Print and shaded views of the part. All mm, measured from the part's lowest x, y and z. Round coordinates to 2 decimals unless told otherwise and drop trailing zeros. Loops run counter-clockwise (first coordinate to the right, second up) from the corner with the lowest first, then second, coordinate; pieces in that order, holes last. Notation, with made-up numbers: (42.25, 84) - (73.25, 84) arc R21 ccw to (73.25, 108) - close; hole circle Ø9 at (27.25, 69). An arc over 180 degrees is marked (long way). Use one line per item in the form item = value.
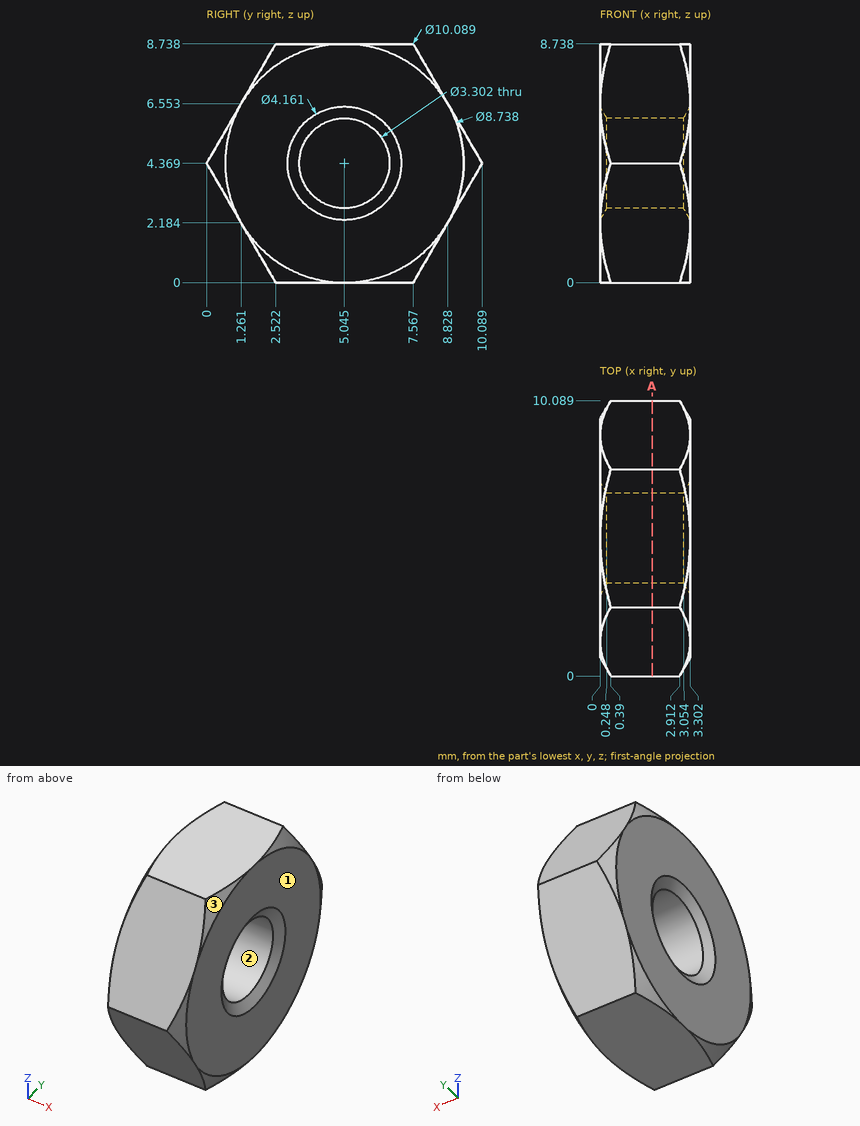
1. Flat gauge pins, fed straight in: pin 1 (1.5 mm diameter, centred on x = 3, z = 1, fed in from -Y); pin 2 (1.5 mm diameter, centred on x = 2, z = 7.5, fed in from +Y) (1 decimal). Where does each tip first touch, or does it go through?
Geometry check:
pin_1 = 1.51
pin_2 = 8.7
2. Pull direction Z, two halves, no side cores. Call the marked faces 1, 2 and 3: +Z half, -Z half, draft (parallel to the pull), parting line (faces both ways), or undercut.
Geometry check:
face_1 = draft
face_2 = undercut
face_3 = +Z half
3. Cut at A-A, the plane x = 1.9. Give the cut face in (y, z) (1 decimal).
Geometry check:
outline = (0, 4.4) - (2.5, 0) - (7.6, 0) - (10.1, 4.4) - (7.6, 8.7) - (2.5, 8.7) - close; hole circle Ø3.3 at (5, 4.4)
4. Wall check: probe 1 along Y at (x, z) = (2.5, 3.5); probe 2 along Z at (x, y) = (2.6, 5.25); probe 3 along Y at (x, z) = (3.1, 5.25) (1 decimal). Give the ranges that are in metal, low to high.
Geometry check:
probe_1 = 0.5 to 3.64, 6.45 to 9.59
probe_2 = 0 to 2.73, 6.01 to 8.74
probe_3 = 0.5 to 3.6, 6.5 to 9.6
